from build123d import *

# Parameters (mm, degrees)
SKETCH1_W           = 150
SKETCH1_H           = 200
BOSS_EXTRUDE1_DEPTH = 30
SKETCH2_W           = 150
SKETCH2_H           = 10
BOSS_EXTRUDE2_DEPTH = 150
SKETCH3_R           = 1.65
SKETCH3_R_2         = 2.25
CUT_EXTRUDE3_DEPTH  = 80
SKETCH6_R           = 5
CUT_EXTRUDE5_DEPTH  = 22
SKETCH7_R           = 1.925
CUT_EXTRUDE6_DEPTH  = 5
FILLET1_R           = 5
SKETCH9_R           = 2.08
CUT_EXTRUDE7_DEPTH  = 30
SKETCH12_W          = 26
SKETCH12_H          = 65
SKETCH12_R          = 2.08
BOSS_EXTRUDE5_DEPTH = 85
SKETCH13_W          = 150
SKETCH13_H          = 60
BOSS_EXTRUDE6_DEPTH = 30
SKETCH15_R          = 2.08
CUT_EXTRUDE8_DEPTH  = 30
SKETCH16_R          = 7
CUT_EXTRUDE9_DEPTH  = 22
SKETCH17_W          = 20
SKETCH17_H          = 260
CUT_EXTRUDE10_DEPTH = 180
SKETCH19_W          = 26
SKETCH19_H          = 65
CUT_EXTRUDE11_DEPTH = 20
SKETCH20_W          = 110
SKETCH20_H          = 12.480627484
CUT_EXTRUDE12_DEPTH = 200
SKETCH21_W          = 10
SKETCH21_H          = 260
CUT_EXTRUDE13_DEPTH = 200
SKETCH22_W          = 21.000744215
SKETCH22_H          = 10
CUT_EXTRUDE14_DEPTH = 80
SKETCH24_W          = 20.877179784
SKETCH24_H          = 9.5
CUT_EXTRUDE15_DEPTH = 25
SKETCH25_R          = 2.25
CUT_EXTRUDE16_DEPTH = 10
SKETCH26_R          = 2.25
CUT_EXTRUDE17_DEPTH = 10
SKETCH27_R          = 2.25
CUT_EXTRUDE18_DEPTH = 10
SKETCH28_R          = 2.25
CUT_EXTRUDE19_DEPTH = 10
SKETCH29_R          = 2.25
CUT_EXTRUDE20_DEPTH = 10
CHAMFER2_SIZE       = 100
CHAMFER2_SIZE2      = 17.632698071
SKETCH33_W          = 40
SKETCH33_H          = 17.63
CUT_EXTRUDE21_DEPTH = 170


with BuildPart() as part:
    # Sketch1 → Boss-Extrude1 (new body)
    with BuildSketch(Plane.XY):
        Rectangle(SKETCH1_W, SKETCH1_H)
    extrude(amount=BOSS_EXTRUDE1_DEPTH)

    # Sketch2 → Boss-Extrude2 (add)
    with BuildSketch(Plane.XY.offset(30)):
        with Locations((0, 95)):
            Rectangle(SKETCH2_W, SKETCH2_H)
    extrude(amount=BOSS_EXTRUDE2_DEPTH)

    # Sketch3 → Cut-Extrude3 (cut)
    with BuildSketch(Plane.XY.offset(30)):
        with Locations((12.5, 46.5)):
            Circle(SKETCH3_R)
        with Locations((-12.5, 46.5)):
            Circle(SKETCH3_R_2)
        with Locations((12.5, 71.5)):
            Circle(SKETCH3_R)
        with Locations((-12.5, 71.5)):
            Circle(SKETCH3_R_2)
    extrude(amount=-CUT_EXTRUDE3_DEPTH, mode=Mode.SUBTRACT)

    # Sketch6 → Cut-Extrude5 (cut)
    with BuildSketch(Plane.XY.offset(30)):
        with Locations((-12.5, 71.5)):
            Circle(SKETCH6_R)
        with Locations((12.5, 71.5)):
            Circle(SKETCH6_R)
        with Locations((-12.5, 46.5)):
            Circle(SKETCH6_R)
        with Locations((12.5, 46.5)):
            Circle(SKETCH6_R)
    extrude(amount=-CUT_EXTRUDE5_DEPTH, mode=Mode.SUBTRACT)

    # Sketch7 → Cut-Extrude6 (cut)
    with BuildSketch(Plane.XY.offset(8)):
        with Locations((-12.5, 71.5)):
            Circle(SKETCH7_R)
        with Locations((12.5, 71.5)):
            Circle(SKETCH7_R)
        with Locations((-12.5, 46.5)):
            Circle(SKETCH7_R)
        with Locations((12.5, 46.5)):
            Circle(SKETCH7_R)
    extrude(amount=-CUT_EXTRUDE6_DEPTH, mode=Mode.SUBTRACT)

    # Fillet1
    fillet1_edges = [part.edges().sort_by_distance(p)[0] for p in [
        (0, 90, 30),
    ]]
    fillet(fillet1_edges, radius=FILLET1_R)

    # Sketch9 → Cut-Extrude7 (cut)
    with BuildSketch(Plane.XY.offset(30)):
        Polygon((-10, -26.5), (-3, -26.5), (-3, 15.5), (-24, 15.5), (-24, -26.5), (-17, -26.5), (-17, -32.5), (-10, -32.5), align=None)
        with Locations((-18.5, 19.25)):
            Circle(SKETCH9_R)
        with Locations((-8.5, 19.25)):
            Circle(SKETCH9_R)
    extrude(amount=-CUT_EXTRUDE7_DEPTH, mode=Mode.SUBTRACT)

    # Sketch12 → Boss-Extrude5 (add)
    with BuildSketch(Plane(origin=(0, 0, 0), x_dir=(-1, 0, 0), z_dir=(0, 0, -1))):
        with Locations((13.5, -4.961410483)):
            Rectangle(SKETCH12_W, SKETCH12_H)
        with Locations((8.5, 19.25)):
            Circle(SKETCH12_R, mode=Mode.SUBTRACT)
        with Locations((18.5, 19.25)):
            Circle(SKETCH12_R, mode=Mode.SUBTRACT)
        Polygon((3, 15.5), (3, -26.5), (10, -26.5), (10, -32.5), (17, -32.5), (17, -26.5), (24, -26.5), (24, 15.5), align=None, mode=Mode.SUBTRACT)
    extrude(amount=-BOSS_EXTRUDE5_DEPTH)

    # Sketch13 → Boss-Extrude6 (add)
    with BuildSketch(Plane(origin=(0, 0, 0), x_dir=(-1, 0, 0), z_dir=(0, 0, -1))):
        with Locations((0, -130)):
            Rectangle(SKETCH13_W, SKETCH13_H)
    extrude(amount=-BOSS_EXTRUDE6_DEPTH)

    # Sketch15 → Cut-Extrude8 (cut)
    with BuildSketch(Plane.XY.offset(30)):
        with Locations((-4.843183012, -101.421536398)):
            Circle(SKETCH15_R)
        with Locations((5.156816988, -101.421536398)):
            Circle(SKETCH15_R)
        Polygon((-10.343183012, -105.171536398), (10.656816988, -105.171536398), (10.656816988, -147.171536398), (3.656816988, -147.171536398), (3.656816988, -153.171536398), (-3.343183012, -153.171536398), (-3.343183012, -147.171536398), (-10.343183012, -147.171536398), align=None)
    extrude(amount=-CUT_EXTRUDE8_DEPTH, mode=Mode.SUBTRACT)

    # Sketch16 → Cut-Extrude9 (cut)
    with BuildSketch(Plane.XY.offset(30)):
        with Locations((-12.5, 71.5)):
            Circle(SKETCH16_R)
        with Locations((12.5, 71.5)):
            Circle(SKETCH16_R)
        with Locations((12.5, 46.5)):
            Circle(SKETCH16_R)
        with Locations((-12.5, 46.5)):
            Circle(SKETCH16_R)
    extrude(amount=-CUT_EXTRUDE9_DEPTH, mode=Mode.SUBTRACT)

    # Sketch17 → Cut-Extrude10 (cut)
    with BuildSketch(Plane(origin=(0, 0, 0), x_dir=(-1, 0, 0), z_dir=(0, 0, -1))):
        with Locations((65, -30)):
            Rectangle(SKETCH17_W, SKETCH17_H)
        with Locations((-65, -30)):
            Rectangle(SKETCH17_W, SKETCH17_H)
    extrude(amount=-CUT_EXTRUDE10_DEPTH, mode=Mode.SUBTRACT)

    # Sketch19 → Cut-Extrude11 (cut)
    with BuildSketch(Plane.XY.offset(30)):
        Polygon((-55, 85), (55, 85), (55, -160), (19, -160), (19, -91.388207499), (-19, -91.388207499), (-19, -160), (-55, -160), align=None)
        with Locations((-13.5, -4.961410483)):
            Rectangle(SKETCH19_W, SKETCH19_H, mode=Mode.SUBTRACT)
    extrude(amount=-CUT_EXTRUDE11_DEPTH, mode=Mode.SUBTRACT)

    # Sketch20 → Cut-Extrude12 (cut)
    with BuildSketch(Plane.XY.offset(10)):
        with Locations((0, 91.240313742)):
            Rectangle(SKETCH20_W, SKETCH20_H)
    extrude(amount=CUT_EXTRUDE12_DEPTH, mode=Mode.SUBTRACT)

    # Sketch21 → Cut-Extrude13 (cut)
    with BuildSketch(Plane(origin=(0, 0, 0), x_dir=(-1, 0, 0), z_dir=(0, 0, -1))):
        with Locations((50, -30)):
            Rectangle(SKETCH21_W, SKETCH21_H)
        with Locations((-50, -30)):
            Rectangle(SKETCH21_W, SKETCH21_H)
    extrude(amount=-CUT_EXTRUDE13_DEPTH, mode=Mode.SUBTRACT)

    # Sketch22 → Cut-Extrude14 (cut)
    with BuildSketch(Plane(origin=(0, 0, 0), x_dir=(-1, 0, 0), z_dir=(0, 0, -1))):
        with Locations((13.500372108, 20.5)):
            Rectangle(SKETCH22_W, SKETCH22_H)
    extrude(amount=-CUT_EXTRUDE14_DEPTH, mode=Mode.SUBTRACT)

    # Sketch24 → Cut-Extrude15 (cut)
    with BuildSketch(Plane(origin=(0, 0, 0), x_dir=(-1, 0, 0), z_dir=(0, 0, -1))):
        with Locations((-0.09540688, -100.421536398)):
            Rectangle(SKETCH24_W, SKETCH24_H)
    extrude(amount=-CUT_EXTRUDE15_DEPTH, mode=Mode.SUBTRACT)

    # Sketch25 → Cut-Extrude16 (cut)
    with BuildSketch(Plane.XY.offset(8)):
        with Locations((12.5, 71.5)):
            Circle(SKETCH25_R)
    extrude(amount=-CUT_EXTRUDE16_DEPTH, mode=Mode.SUBTRACT)

    # Sketch26 → Cut-Extrude17 (cut)
    with BuildSketch(Plane.XY.offset(8)):
        with Locations((12.5, 46.5)):
            Circle(SKETCH26_R)
    extrude(amount=-CUT_EXTRUDE17_DEPTH, mode=Mode.SUBTRACT)

    # Sketch27 → Cut-Extrude18 (cut)
    with BuildSketch(Plane.XY.offset(85)):
        with Locations((-18.5, 19.25)):
            Circle(SKETCH27_R)
    extrude(amount=-CUT_EXTRUDE18_DEPTH, mode=Mode.SUBTRACT)

    # Sketch28 → Cut-Extrude19 (cut)
    with BuildSketch(Plane.XY.offset(85)):
        with Locations((-8.5, 19.25)):
            Circle(SKETCH28_R)
    extrude(amount=-CUT_EXTRUDE19_DEPTH, mode=Mode.SUBTRACT)

    # Sketch29 → Cut-Extrude20 (cut)
    with BuildSketch(Plane.XY.offset(30)):
        with Locations((-4.843183012, -101.421536398)):
            Circle(SKETCH29_R)
        with Locations((5.156816988, -101.421536398)):
            Circle(SKETCH29_R)
    extrude(amount=-CUT_EXTRUDE20_DEPTH, mode=Mode.SUBTRACT)

    # Chamfer2
    chamfer2_edges = [part.edges().sort_by_distance(p)[0] for p in [
        (0, 97.480627484, 10),
    ]]
    chamfer2_side = [part.faces().sort_by_distance(p)[0] for p in [
        (0, 97.480627484, 95),
    ]]
    chamfer(chamfer2_edges, length=CHAMFER2_SIZE, length2=CHAMFER2_SIZE2, reference=chamfer2_side[0])

    # Sketch33 → Cut-Extrude21 (cut)
    with BuildSketch(Plane.XY.offset(10)):
        with Locations((-20, 88.662929413)):
            Rectangle(SKETCH33_W, SKETCH33_H)
        with Locations((20, 88.662929413)):
            Rectangle(SKETCH33_W, SKETCH33_H)
    extrude(amount=CUT_EXTRUDE21_DEPTH, mode=Mode.SUBTRACT)


solid = part.part
Model file for the job. Use its own axes, mm. A direction names the side the tool comes from. Round coordinates to 2 decimals unless told otherwise and drop trailing zeros. Order: outer loops, then holes, each group sorted by start corner. A loop starts at its lowest first (then second) coordinate and runs counter-clockwise, first axis right, second up.
(1) Drill centre lines: line 1 (Y direction, x = -12.5, z = 9.4); line 2 (Y direction, x = 12.5, z = 9); line 3 (Y direction, x = -12, z = 4). Where is each one in solid material? Low to high.
(2) Band-saw the part on A-A (y = -19). List the corners of the cut face in (x, z), then the cut area to 4 significant figures.
(3) Pin check, flat tips, straight feed: pin 1 (4 mm diameter, centred on y = -3, z = 50, fed in from -X); pin 2 (10 mm diameter, centred on y = -120.5, z = 20.5, fed in from -X); pin 3 (1 mm diameter, centred on x = 29, z = 94, fed in from -Y). Stop position of each tip, or through.
(4) Band-saw the part on D-D (y = -125). List the corners of the cut face in (x, z), then the cut area to 3 significant figures.
(5) Band-saw the part on C-C (z = 115). List the corners of the cut face in (x, y).
(6) Pull direction Y, two halves, no side cores. Call faces 4 (the face through (-19, -125, 20)), 5 (the face through (-40.21, 88.623, 59.767)), 6 (the face through (-13, 15.5, 83)): released by +Y, released by -Y, zero draft, split by the parting line, or undercut.
(7) 3-axis set-ups, long thin cutter, end or side, ignore diameter. For faces 1 (the face through (10.657, -126, 15)), 2 (the face through (-14, 27.539, 48)), 3 (the face through (-13, 25.5, 39)): which of +Z, -Z, +X, -X, +Y, -Y reach the whole face in a straight line?
Verdict:
1. line 1: y = -160 to -32.5, 25.5 to 39.5, 53.5 to 64.5, 78.5 to 100
1. line 2: y = -160 to 39.5, 53.5 to 64.5, 78.5 to 100
1. line 3: y = -160 to -32.5, 25.5 to 44.31, 48.69 to 69.31, 73.69 to 100
2. outline: (-45, 0) - (-24, 0) - (-24, 85) - (-26.5, 85) - (-26.5, 10) - (-45, 10) - close; (-3, 0) - (45, 0) - (45, 10) - (-0.5, 10) - (-0.5, 85) - (-3, 85) - close
2. area: 1,065 mm2
3. pin 1: stops at x = -26.5
3. pin 2: stops at x = -19
3. pin 3: stops at y = 97.48
4. outline: (-45, 0) - (-10.34, 0) - (-10.34, 30) - (-19, 30) - (-19, 10) - (-45, 10) - close; (10.66, 0) - (45, 0) - (45, 10) - (19, 10) - (19, 30) - (10.66, 30) - close
4. area: 1,030 mm2
5. outline: (-45, 97.48) - (45, 97.48) - (45, 100) - (-45, 100) - close
6. face 4: zero draft
6. face 5: released by -Y
6. face 6: undercut
7. face 1: +Z, -Z
7. face 2: +Z, +X, -X
7. face 3: -Z
